Geometry: final body of the model. Coordinates: model frame, mm. Face numbers are marked on the shaded views. A direction names the side the tool comes from. Round coordinates to 2 decimals unless told otherwise and drop trailing zeros. Loops run counter-clockwise (first coordinate to the right, second up) from the corner with the lowest first, then second, coordinate; pieces in that order, holes last. Notation, with made-up numbers: (17.5, 71.5) -> (62.5, 71.5) arc R22 cw to (62.5, 110.5) -> close; hole circle Ø11 at (-32.75, 67). An arc over 180 degrees is marked (long way). Answer in a Markdown table with one row per item.
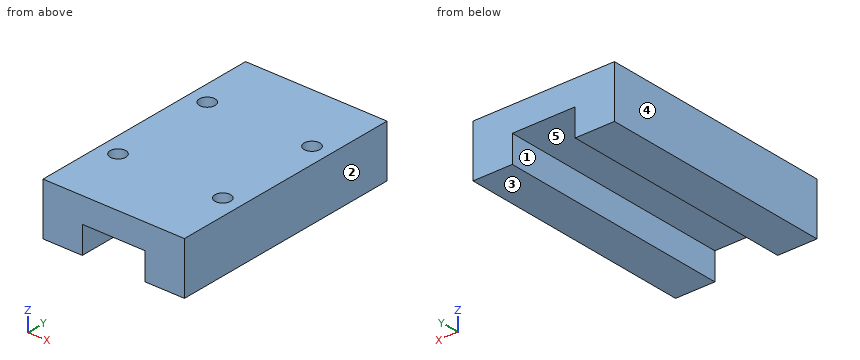
Autodesk Inventor part; units mm, degrees
sketch "Эскиз1" plane through (0, 0, 0) normal (0, 1, 0) x (-1, 0, 0)
  line L0 (-13.5, -5) -> (13.5, -5)
  line L1 (13.5, -5) -> (13.5, 5)
  line L2 (13.5, 5) -> (-13.5, 5)
  line L3 (-13.5, 5) -> (-13.5, -5)
  line L4 (-13.5, -5) -> (13.5, 5) construction
  line L5 (13.5, -5) -> (-13.5, 5) construction
  line L6 (-6, -5) -> (6, -5)
  line L7 (6, -5) -> (6, 0.2)
  line L8 (6, 0.2) -> (-6, 0.2)
  line L9 (-6, 0.2) -> (-6, -5)
  line L10 (0, -7) -> (0, 7) construction
  point P0 (0, 0)
  point P1 (0, 0.2)
  dimension "d0" = 27
  dimension "d1" = 10
  dimension "d2" = 12
  dimension "d3" = 5.2
extrude "Выдавливание1" add sketch "Эскиз1" along normal mid plane 45.4 contours L3 L2 L1 L0 L7 L8 L9
sketch "Эскиз2" plane through (-13.5, 22.7, 5) normal (0, 0, 1) x (1, 0, 0)
  circle A0 centre (3.5, -12.7) radius 1.5
  circle A1 centre (3.5, -32.7) radius 1.5
  circle A2 centre (23.5, -12.7) radius 1.5
  circle A3 centre (23.5, -32.7) radius 1.5
  line L0 (3.5, -12.7) -> (3.5, -32.7) construction
  line L1 (3.5, -32.7) -> (23.5, -12.7) construction
  line L2 (23.5, -12.7) -> (3.5, -12.7) construction
  line L3 (23.5, -32.7) -> (23.5, -12.7) construction
  line L4 (3.5, -32.7) -> (23.5, -32.7) construction
  line L5 (23.5, -32.7) -> (3.5, -12.7) construction
  point P0 (13.5, -22.7)
  point P1 (13.5, -22.7)
  dimension "d6" = 3
  dimension "d7" = 20
  dimension "d8" = 20
extrude "Выдавливание2" cut sketch "Эскиз2" against normal blind 5
properties part number "Каретка"
Item 1: Ray query, L1, parallel to Y at x = -10, z = 3.1; L2, parallel to X at y = 1.5, z = -0.5; L3, parallel to Y at x = 11.25, z = 3.75. Return the intervals inside material, ascending.
Ans:
| item | result |
|---|---|
| L1 | -22.7 to -11.5, -8.5 to 8.5, 11.5 to 22.7 |
| L2 | -13.5 to -6, 6 to 13.5 |
| L3 | -22.7 to -10.83, -9.17 to 9.17, 10.83 to 22.7 |
Item 2: Section query A-A, the plane y = -10. Output: boundary loops of the cut face in (x, z).
Ans:
| item | result |
|---|---|
| outline | (-13.5, -5) -> (-6, -5) -> (-6, 0.2) -> (6, 0.2) -> (6, -5) -> (13.5, -5) -> (13.5, 5) -> (11.5, 5) -> (11.5, 0) -> (8.5, 0) -> (8.5, 5) -> (-8.5, 5) -> (-8.5, 0) -> (-11.5, 0) -> (-11.5, 5) -> (-13.5, 5) -> close |
Item 3: Set-up query: the marked faces 1 and 2. Return all of +Z, -Z, +X, -X, +Y, -Y with unobstructed straight access to the full face (end or side cutting, diameter ignored); none if empty.
Ans:
| item | result |
|---|---|
| face 1 | -Z, +Y, -Y |
| face 2 | +Z, -Z, +X, +Y, -Y |
Item 4: Section query B-B, the plane x = -10. Output: boundary loops of the cut face in (y, z), and give its area (3 significant figures).
Ans:
| item | result |
|---|---|
| outline | (-22.7, -5) -> (22.7, -5) -> (22.7, 5) -> (11.5, 5) -> (11.5, 0) -> (8.5, 0) -> (8.5, 5) -> (-8.5, 5) -> (-8.5, 0) -> (-11.5, 0) -> (-11.5, 5) -> (-22.7, 5) -> close |
| area | 424 mm2 |
Item 5: Section query C-C, the plane x = 0.5. Output: boundary loops of the cut face in (y, z), and give its area (3 significant figures).
Ans:
| item | result |
|---|---|
| outline | (-22.7, 0.2) -> (22.7, 0.2) -> (22.7, 5) -> (-22.7, 5) -> close |
| area | 218 mm2 |
Item 6: Section query D-D, the plane x = 10.5. Output: boundary loops of the cut face in (y, z), and give its area (3 significant figures).
Ans:
| item | result |
|---|---|
| outline | (-22.7, -5) -> (22.7, -5) -> (22.7, 5) -> (11.41, 5) -> (11.41, 0) -> (8.59, 0) -> (8.59, 5) -> (-8.59, 5) -> (-8.59, 0) -> (-11.41, 0) -> (-11.41, 5) -> (-22.7, 5) -> close |
| area | 426 mm2 |
Item 7: First-contact query: P1, Ø0.9, axis at x = 9.5, y = 9.5, coming from the +Z side; P2, Ø6, axis at x = 0.5, y = -4, coming from the -Z side. Flat tips, straight axial feed; report the tip coordinate or a pass-through.
Ans:
| item | result |
|---|---|
| P1 | z = 0 |
| P2 | z = 0.2 |
Item 8: Mould query, pull axis X, two halves, no side actions, for the marked faces 3, 4 and 5. Classes: released by +X, released by -X, zero draft, split by the parting line, or undercut.
Ans:
| item | result |
|---|---|
| face 3 | zero draft |
| face 4 | released by -X |
| face 5 | undercut |
